Geometry: final body of the model. Coordinates: model frame, mm. A direction names the side the tool comes from. Coordinates: 2 decimals unless noted, no trailing zeros. Write each loop counter-clockwise with the first axis right and the second up, starting at its lowest first coordinate (ties: lowest second). Pieces come first, ordered by that corner, then holes. Notation, with made-up numbers: (-6, 55.25) -> (28, 55.25) arc R27 cw to (28, 85.25) -> close; hole circle Ø5 at (-25.75, 33). An arc over 180 degrees is marked (long way). Answer as a JSON object with one key per item and string values. Group by question number.
```python
from build123d import *

# Parameters (mm, degrees)
BOSS_EXTRU_2_DEPTH   = 50
R_SERVOIR_TEST_3_W   = 15
R_SERVOIR_TEST_3_H   = 15
BOSS_EXTRU_3_DEPTH   = 5
D_GAGEMENT_M41_D     = 4.5
D_GAGEMENT_M41_DEPTH = 5
D_GAGEMENT_M41_TIP   = 1.351936393
COQUE3_START         = 2
COQUE3_OUTLINE_W     = 116
COQUE3_OUTLINE_H     = 46
COQUE3_DEPTH         = 46
COQUE3_2_OUTLINE_W   = 15
COQUE3_2_OUTLINE_H   = 11
COQUE3_2_OUTLINE_R   = 4.25
COQUE3_2_DEPTH       = 1


# Read off the part's stored shape, not the designer's step: Coque3
with BuildPart() as part:
    # Réservoir test → Boss.-Extru.2 (new body)
    with BuildSketch(Plane(origin=(0, 0, 0), x_dir=(1, 0, 0), z_dir=(0, 1, 0))):
        Polygon((60, 0), (60, 50), (0, 50), (0, 32.5), (0, 17.5), (0, 0), align=None)
        Polygon((120, 50), (60, 50), (60, 0), (120, 0), (120, 17.5), (120, 32.5), align=None)
    extrude(amount=BOSS_EXTRU_2_DEPTH)

    # Réservoir test<3> → Boss.-Extru.3 (add)
    with BuildSketch(Plane(origin=(0, 0, 0), x_dir=(1, 0, 0), z_dir=(0, 1, 0))):
        with Locations((-7.5, 25)):
            Rectangle(R_SERVOIR_TEST_3_W, R_SERVOIR_TEST_3_H)
        with Locations((127.5, 25)):
            Rectangle(R_SERVOIR_TEST_3_W, R_SERVOIR_TEST_3_H)
    extrude(amount=BOSS_EXTRU_3_DEPTH)

    # Dégagement M41
    with Locations(Plane(origin=(0, 5, 0), x_dir=(1, 0, 0), z_dir=(0, 1, 0))):
        with Locations((-7.5, 25), (127.5, 25)):
            Hole(D_GAGEMENT_M41_D / 2, depth=D_GAGEMENT_M41_DEPTH)
            with Locations((0, 0, -(D_GAGEMENT_M41_DEPTH + D_GAGEMENT_M41_TIP / 2))):  # 118° drill point
                Cone(0, D_GAGEMENT_M41_D / 2, D_GAGEMENT_M41_TIP, mode=Mode.SUBTRACT)

    # Coque3 outline → Coque3 (cut)
    with BuildSketch(Plane(origin=(0, 0, 0), x_dir=(1, 0, 0), z_dir=(0, 1, 0)).offset(COQUE3_START)):
        with Locations((60, 25)):
            Rectangle(COQUE3_OUTLINE_W, COQUE3_OUTLINE_H)
    extrude(amount=COQUE3_DEPTH, mode=Mode.SUBTRACT)

    # Coque3 2 outline → Coque3 2 (cut)
    # profile 1 of 2: a face of its own
    with BuildSketch(Plane(origin=(0, 0, 0), x_dir=(1, 0, 0), z_dir=(0, 1, 0)).offset(COQUE3_START)):
        with Locations((125.5, 25)):
            Rectangle(COQUE3_2_OUTLINE_W, COQUE3_2_OUTLINE_H)
        with Locations((127.5, 25)):
            Circle(COQUE3_2_OUTLINE_R, mode=Mode.SUBTRACT)
    # profile 2 of 2: a face of its own
    with BuildSketch(Plane(origin=(0, 0, 0), x_dir=(1, 0, 0), z_dir=(0, 1, 0)).offset(COQUE3_START)):
        with Locations((-5.5, 25)):
            Rectangle(COQUE3_2_OUTLINE_W, COQUE3_2_OUTLINE_H)
        with Locations((-7.5, 25)):
            Circle(COQUE3_2_OUTLINE_R, mode=Mode.SUBTRACT)
    extrude(amount=COQUE3_2_DEPTH, mode=Mode.SUBTRACT)


solid = part.part
```
Item 1: Section A-A on z = -25. Give the number of separate pieces and of enclosed holes in the cut face, then the cut area to 3 significant figures.
Item 2: Mould query, pull axis Z, two halves, no side actions, for faces 1 (the flat face through (59, 25, -48)), 2 (the flat face through (2, 25, -25)), 3 (the flat face through (59, 25, 0)), 4 (the flat face through (59, 50, -25)). Classes: +Z half, -Z half, draft (parallel to the pull), parting line (faces both ways), or undercut.
Item 3: Contact query for flat-ended pins moving along their axis: pin 1 (1.5 mm diameter, centred on x = 129, y = 2.5, fed in from -Z); pin 2 (5.5 mm diameter, centred on x = 129.5, y = 2.5, fed in from +Z); pin 3 (4 mm diameter, centred on y = 18.5, z = -13, fed in from +X). Output: stop coordinate, or through.
Item 4: Section C-C on y = 26.5. Output: boundary loops of the cut face in (x, z).
Item 5: Set-up query: faces 5 (the flat face through (-8, 2, -32.5)), 6 (the cylindrical face through (123.254, 2.493, -25.187)), 7 (the flat face through (126, 5, -27)). Return all of +Z, -Z, +X, -X, +Y, -Y with unobstructed straight access to the full face (end or side cutting, diameter ignored); none if empty.
Item 6: Section D-D on z = -3.5. Output: boundary loops of the cut face in (x, y).
Item 7: Ray query, L1, parallel to Z at x = 127.5, y = 2.3; L2, parallel to X at y = 31, z = -17.5; L3, parallel to X at y = 1, z = -25. Return the intervals inside material, ascending. Write a range as [from, to].
Item 8: Section B-B on x = 127.5. Output: boundary loops of the cut face in (y, z).
Answer sheet:
{
 "1": {"separate pieces": "3", "enclosed holes": "3", "area": "756 mm^2"},
 "2": {"face 1": "undercut", "face 2": "undercut", "face 3": "+Z half", "face 4": "draft"},
 "3": {"pin 1": "stops at z = -32.5", "pin 2": "stops at z = -17.5", "pin 3": "stops at x = 120"},
 "4": {"outline": "(0, -50) -> (120, -50) -> (120, 0) -> (0, 0) -> close; hole (2, -48) -> (118, -48) -> (118, -2) -> (2, -2) -> close"},
 "5": {"face 5": "-Z, -X, +Y, -Y", "face 6": "none", "face 7": "+Z, -Z, +X, +Y"},
 "6": {"outline": "(0, 0) -> (120, 0) -> (120, 50) -> (0, 50) -> close; hole (2, 2) -> (118, 2) -> (118, 48) -> (2, 48) -> close"},
 "7": {"L1": "z = [-32.5, -30.5], [-29.25, -27.25], [-22.75, -20.75], [-19.5, -17.5]", "L2": "x = [0, 2], [118, 120]", "L3": "x = [-15, -9.75], [-5.25, 125.25], [129.75, 135]"},
 "8": {"outline": "(0, -32.5) -> (5, -32.5) -> (5, -27.25) -> (0, -27.25) -> close; (0, -22.75) -> (5, -22.75) -> (5, -17.5) -> (0, -17.5) -> close; hole (2, -30.5) -> (3, -30.5) -> (3, -29.25) -> (2, -29.25) -> close; hole (2, -20.75) -> (3, -20.75) -> (3, -19.5) -> (2, -19.5) -> close"}
}
